Input: dimensioned drawing with shaded views. Units: mm. Origin: part minimum x, y, z. Coordinates: 2 decimals unless noted, no trailing zeros. Loops run counter-clockwise (first coordinate to the right, second up) from the corner with the lowest first, then second, coordinate; pieces in that order, holes last. Notation, with made-up numbers: (63.5, -11) - (122.5, -11) arc R7 ccw to (122.5, -3) - close; hole circle Ø3 at (68.5, 74.25). An arc over 180 degrees is marked (long way). Write item = value, one per line. Start each with the question number.
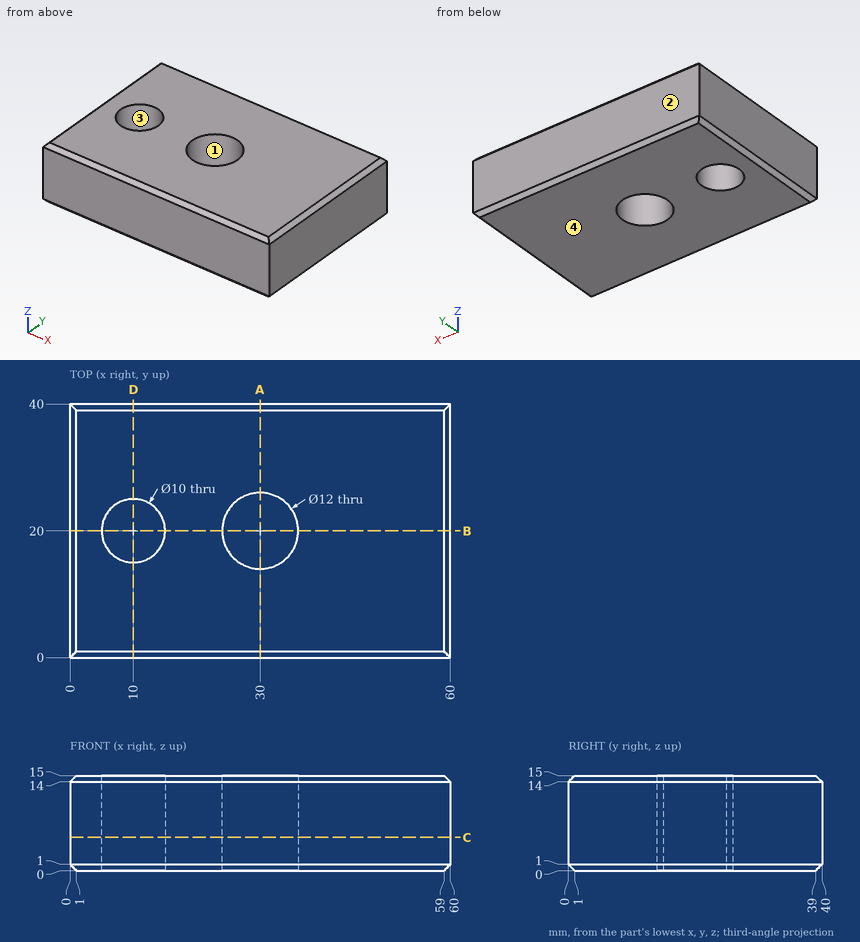
Item 1: Cut plane D-D on x = 10. Return loops of the section in (y, z).
Item 2: Cut plane A-A on x = 30. Return loops of the section in (y, z), plus the area to 3 significant figures.
Item 3: Cut plane B-B on y = 20. Return loops of the section in (x, z).
Item 4: Pull-direction query (Y, two-part tool) for the marked faces 1, 2, 3 and 4; classes: pulls with the +Y half, pulls with the -Y half, needs draft (parallel to the pull), parting line crosses it, or undercut.
Item 5: Cut plane C-C on z = 5.25. Return loops of the section in (x, y).
Item 6: Ray query, line 1 (Y direction, x = 30, z = 9.75); line 2 (X direction, y = 21, z = 9); line 3 (X direction, y = 17, z = 11). Return the intervals inside material, ascending.
Recorded:
q1.outline = (0, 1) - (1, 0) - (15, 0) - (15, 15) - (1, 15) - (0, 14) - close; (25, 0) - (39, 0) - (40, 1) - (40, 14) - (39, 15) - (25, 15) - close
q2.outline = (0, 1) - (1, 0) - (14, 0) - (14, 15) - (1, 15) - (0, 14) - close; (26, 0) - (39, 0) - (40, 1) - (40, 14) - (39, 15) - (26, 15) - close
q2.area = 418 mm²
q3.outline = (0, 1) - (1, 0) - (5, 0) - (5, 15) - (1, 15) - (0, 14) - close; (15, 0) - (24, 0) - (24, 15) - (15, 15) - close; (36, 0) - (59, 0) - (60, 1) - (60, 14) - (59, 15) - (36, 15) - close
q4.face_1 = undercut
q4.face_2 = pulls with the +Y half
q4.face_3 = undercut
q4.face_4 = needs draft
q5.outline = (0, 0) - (60, 0) - (60, 40) - (0, 40) - close; hole circle Ø10 at (10, 20); hole circle Ø12 at (30, 20)
q6.line_1 = 0 to 14, 26 to 40
q6.line_2 = 0 to 5.1, 14.9 to 24.08, 35.92 to 60
q6.line_3 = 0 to 6, 14 to 24.8, 35.2 to 60
